```python
from build123d import *

# Parameters (mm, degrees)
SKETCH1_R                = 0.9
SKETCH1_R_2              = 0.5
SKETCH1_W                = 1
SKETCH1_H                = 0.5
BOSS_EXTRUDE1_DEPTH      = 1
BOSS_EXTRUDE2_DEPTH      = 11
BOSS_EXTRUDE2_DEPTH_BACK = 1.2
SKETCH2_R                = 0.5
SKETCH2_R_2              = 0.25
SKETCH3_R                = 0.66091417
CUT_EXTRUDE3_DEPTH       = 0.1
SKETCH4_R                = 0.55
CUT_EXTRUDE4_DEPTH       = 10.9
SKETCH5_R                = 0.15
CUT_EXTRUDE5_DEPTH       = 10.9
SCALE1_SCALE             = 10


with BuildPart() as part:
    # Sketch1 → Boss-Extrude1 (new body)
    # profile 1 of 3: a face of its own
    with BuildSketch(Plane.XY):
        Circle(SKETCH1_R)
        Circle(SKETCH1_R_2, mode=Mode.SUBTRACT)
    # profile 2 of 3: a face of its own
    with BuildSketch(Plane.XY):
        with Locations((1.05, 0.25)):
            Rectangle(SKETCH1_W, SKETCH1_H)
    # profile 3 of 3: a face of its own
    with BuildSketch(Plane.XY):
        with Locations((-1.05, 0.25)):
            Rectangle(SKETCH1_W, SKETCH1_H)
    extrude(amount=BOSS_EXTRUDE1_DEPTH)

    # Sketch2 → Boss-Extrude2 (add, two sides: drawn at the far end of the back side and taken through both)
    with BuildSketch(Plane.XY.offset(1).offset(-BOSS_EXTRUDE2_DEPTH_BACK)):
        with Locations((-0.008750419, 0)):
            Circle(SKETCH2_R)
        Circle(SKETCH2_R_2, mode=Mode.SUBTRACT)
    extrude(amount=BOSS_EXTRUDE2_DEPTH + BOSS_EXTRUDE2_DEPTH_BACK)

    # Sketch3 → Cut-Extrude3 (cut)
    with BuildSketch(Plane(origin=(0, 0, -0.2), x_dir=(-1, 0, 0), z_dir=(0, 0, -1))):
        with Locations((0.008750419, 0)):
            Circle(SKETCH3_R)
    extrude(amount=-CUT_EXTRUDE3_DEPTH, mode=Mode.SUBTRACT)

    # Sketch4 → Cut-Extrude4 (cut)
    with BuildSketch(Plane.XY.offset(12)):
        Circle(SKETCH4_R)
    extrude(amount=-CUT_EXTRUDE4_DEPTH, mode=Mode.SUBTRACT)

    # Sketch5 → Cut-Extrude5 (cut)
    with BuildSketch(Plane(origin=(0, 0.5, 0), x_dir=(1, 0, 0), z_dir=(0, 1, 0))):
        with Locations(Location((1.15, -0.5, 0), (0, 0, 270))):
            Circle(SKETCH5_R)
        with Locations(Location((-1.15, -0.5, 0), (0, 0, 270))):
            Circle(SKETCH5_R)
    extrude(amount=-CUT_EXTRUDE5_DEPTH, mode=Mode.SUBTRACT)


with BuildPart() as part_1:
    # Scale1: scaled about (0, 0, 0)
    add(part.part.scale(SCALE1_SCALE))


solid = part_1.part
```
Build history of the part. All positions in model axes, mm. A direction names the side the tool comes from. Round coordinates to 2 decimals unless told otherwise and drop trailing zeros. Order: outer loops, then holes, each group sorted by start corner. A loop starts at its lowest first (then second) coordinate and runs counter-clockwise, first axis right, second up. Notation, with made-up numbers: (-11.5, 10) -> (13.5, 10) arc R24 cw to (13.5, 44) -> close; hole circle Ø8 at (-32, 2). An arc over 180 degrees is marked (long way). Answer in a Markdown table with one row per item.
1) Which spindle directions (+Z, -Z, +X, -X, +Y, -Y) get a long thin tool onto all of the face, cutting with end or side? Do faces 5 (the flat face through (3.2, 4.1, 0)), 6 (the flat face through (3.2, 4.1, 10)), 7 (the flat face through (-13, 0, 4)). Say none if no direction does.
Values:
| item | result |
|---|---|
| face 5 | -Z |
| face 6 | +Z |
| face 7 | +Z, -Z, -X, -Y |
2) Mould opens along Y. For faces 1 (the flat face through (13, 0, 6)), 2 (the cylindrical face through (-0.54, -2.44, 4.92)), 3 (the flat face through (-2.4, 1.2, 11)), 4 (the flat face through (9.7, 5, 4.9)) say: released by +Y, released by -Y, zero draft, split by the parting line, or undercut.
Values:
| item | result |
|---|---|
| face 1 | released by -Y |
| face 2 | undercut |
| face 3 | zero draft |
| face 4 | released by +Y |
3) Pin check, flat tips, straight feed: P1, Ø5, axis at x = 3.5, y = 4.5, coming from the -Z side; P2, Ø1.5, axis at y = -4.5, z = 1, coming from the -X side; P3, Ø2.5, axis at x = 10.5, z = 5, coming from the +Y side; P4, Ø7, axis at x = -13, z = 6.5, coming from the -Y side. Stop position of each tip, or through.
Values:
| item | result |
|---|---|
| P1 | z = -1 |
| P2 | x = -8.18 |
| P3 | y = 5 |
| P4 | y = 0 |
4) Wall check: L1, parallel to Y at x = 14, z = 1; L2, parallel to Z at x = -7, y = 2.5; L3, parallel to X at y = -6.5, z = 3.75. Give the ranges that are in metal, low to high.
Values:
| item | result |
|---|---|
| L1 | 0 to 5 |
| L2 | 0 to 10 |
| L3 | -6.22 to 6.22 |
5) Band-saw the part on C-C on x = 11.5. Give the cut face in (y, z), and give its area (3 significant figures).
Values:
| item | result |
|---|---|
| outline | (0, 0) -> (5, 0) -> (5, 3.5) -> (0, 3.5) -> close; (0, 6.5) -> (5, 6.5) -> (5, 10) -> (0, 10) -> close |
| area | 35.0 mm2 |
6) Band-saw the part on B-B on z = 5.5. Give the cut face in (x, y).
Values:
| item | result |
|---|---|
| outline | (-15.5, 0) -> (-12.91, 0) -> (-12.91, 5) -> (-15.5, 5) -> close; (-10.09, 0) -> (-9, 0) arc R9 ccw to (9, 0) -> (10.09, 0) -> (10.09, 5) -> (7.48, 5) arc R9 ccw to (-7.48, 5) -> (-10.09, 5) -> close; (12.91, 0) -> (15.5, 0) -> (15.5, 5) -> (12.91, 5) -> close; hole circle Ø5 at (0, 0); hole (-0.04, -5) arc R5 ccw (long way) to (-0.04, 5) arc R5 cw to start |
7) Band-saw the part on D-D on y = 1.75. Give the cut face in (x, z), and give its area (3 significant figures).
Values:
| item | result |
|---|---|
| outline | (-15.5, 0) -> (-4.77, 0) -> (-4.77, -1) -> (-1.79, -1) -> (-1.79, 11) -> (-4.77, 11) -> (-4.77, 10) -> (-15.5, 10) -> close; (1.79, -1) -> (4.6, -1) -> (4.6, 11) -> (1.79, 11) -> close; (4.68, 0) -> (15.5, 0) -> (15.5, 10) -> (4.68, 10) -> close; hole circle Ø3 at (-11.5, 5); hole circle Ø3 at (11.5, 5) |
| area | 271 mm2 |
8) Band-saw the part on A-A on y = 4. Give the cut face in (x, z).
Values:
| item | result |
|---|---|
| outline | (-15.5, 0) -> (-3.09, 0) -> (-3.09, -1) -> (2.91, -1) -> (2.91, 11) -> (-3.09, 11) -> (-3.09, 10) -> (-15.5, 10) -> close; (3, 0) -> (15.5, 0) -> (15.5, 10) -> (3, 10) -> close; hole circle Ø3 at (-11.5, 5); hole circle Ø3 at (11.5, 5) |
